Print and shaded views of the part. All mm, measured from the part's lowest x, y and z. Round coordinates to 2 decimals unless told otherwise and drop trailing zeros. Loops run counter-clockwise (first coordinate to the right, second up) from the corner with the lowest first, then second, coordinate; pieces in that order, holes last. Notation, with made-up numbers: (87, 46) - (105, 46) arc R23 cw to (105, 60) - close; hole circle Ø3 at (37.25, 17.5). An arc over 180 degrees is marked (long way). Put each result on its own line as item: value. Start each with the question number.
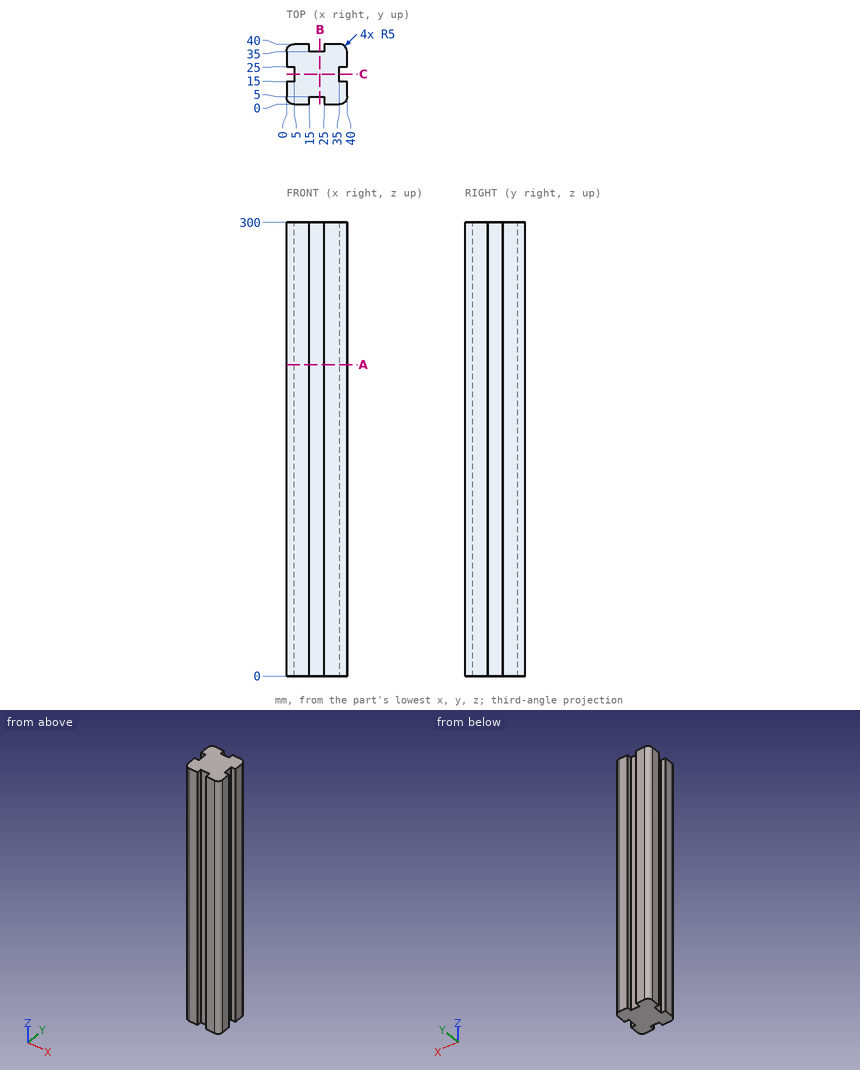
Item 1: Drill centre lines: probe 1 along X at (y, z) = (4.5, 110.5); probe 2 along Y at (x, z) = (3.5, 155); probe 3 along X at (y, z) = (37.5, 142). Where is each one in solid material? Low to high. Write a range as [from, to].
Item 2: Slice it at A-A (z = 206). Give the cut face in (x, y), plus the area to 3 significant figures.
Item 3: Slice it at B-B (x = 22). Give the cut face in (y, z).
Item 4: Drop flat-ended pins along their axis: pin 1 Ø8 at (x, z) = (19.5, 203.5) entering from -Y; pin 2 Ø2.5 at (y, z) = (2, 200.5) entering from +X; pin 3 Ø1.5 at (y, z) = (38.5, 142) entering from -X. Give the stop position or say it passes through.
Computed values:
1. probe 1: x = [0.03, 15], [25, 39.97]
1. probe 2: y = [0.23, 15], [25, 39.77]
1. probe 3: x = [0.67, 15], [25, 39.33]
2. outline: (0, 5) arc R5 ccw to (5, 0) - (15, 0) - (15, 5) - (25, 5) - (25, 0) - (35, 0) arc R5 ccw to (40, 5) - (40, 15) - (35, 15) - (35, 25) - (40, 25) - (40, 35) arc R5 ccw to (35, 40) - (25, 40) - (25, 35) - (15, 35) - (15, 40) - (5, 40) arc R5 ccw to (0, 35) - (0, 25) - (5, 25) - (5, 15) - (0, 15) - close
2. area: 1,380 mm^2
3. outline: (5, 0) - (35, 0) - (35, 300) - (5, 300) - close
4. pin 1: stops at y = 5
4. pin 2: stops at x = 39.68
4. pin 3: stops at x = 0.82
